from build123d import *

# Parameters (mm, degrees)
BOSS_EXTRUDE1_DEPTH   = 42.37
SKETCH2_R             = 7.45
BOSS_EXTRUDE2_DEPTH   = 1.28
BOSS_EXTRUDE3_DEPTH   = 13.58
SKETCH4_W             = 4.9
SKETCH4_H             = 11.6
BOSS_EXTRUDE4_DEPTH   = 3
M2_TAPPED_HOLE1_D     = 1.6
M2_TAPPED_HOLE1_DEPTH = 4
M2_TAPPED_HOLE1_TIP   = 0.480688495


with BuildPart() as part:
    # Sketch1 → Boss-Extrude1 (new body)
    with BuildSketch(Plane.XY):
        with BuildLine():
            Line((-8, -10), (8, -10))
            ThreePointArc((8, -10), (9.414213562, -9.414213562), (10, -8))
            Line((10, -8), (10, 8))
            ThreePointArc((10, 8), (9.414213562, 9.414213562), (8, 10))
            Line((8, 10), (-8, 10))
            ThreePointArc((-8, 10), (-9.414213562, 9.414213562), (-10, 8))
            Line((-10, 8), (-10, -8))
            ThreePointArc((-10, -8), (-9.414213562, -9.414213562), (-8, -10))
        make_face()
    extrude(amount=BOSS_EXTRUDE1_DEPTH)

    # Sketch2 → Boss-Extrude2 (add)
    with BuildSketch(Plane.XY.offset(42.37)):
        with Locations(Location((0, 0, 0), (0, 0, 180))):
            Circle(SKETCH2_R)
    extrude(amount=BOSS_EXTRUDE2_DEPTH)

    # Sketch3 → Boss-Extrude3 (add)
    with BuildSketch(Plane.XY.offset(43.65)):
        with BuildLine():
            Line((-1.5, 1.322875656), (-1.5, -1.322875656))
            ThreePointArc((-1.5, -1.322875656), (2, 0), (-1.5, 1.322875656))
        make_face()
    extrude(amount=BOSS_EXTRUDE3_DEPTH)

    # Sketch4 → Boss-Extrude4 (add)
    with BuildSketch(Plane.ZY.offset(10)):
        with Locations((5.45, 0)):
            Rectangle(SKETCH4_W, SKETCH4_H)
    extrude(amount=BOSS_EXTRUDE4_DEPTH)

    # M2 Tapped Hole1
    with Locations(Plane.XY.offset(42.37)):
        with Locations((-8, -8), (8, -8), (8, 8), (-8, 8)):
            Hole(M2_TAPPED_HOLE1_D / 2, depth=M2_TAPPED_HOLE1_DEPTH)
            with Locations((0, 0, -(M2_TAPPED_HOLE1_DEPTH + M2_TAPPED_HOLE1_TIP / 2))):  # 118° drill point
                Cone(0, M2_TAPPED_HOLE1_D / 2, M2_TAPPED_HOLE1_TIP, mode=Mode.SUBTRACT)


solid = part.part
Input: part model. Units: mm. Frame: model coordinates. A direction names the side the tool comes from. Coordinates: 2 decimals unless noted, no trailing zeros. Write each loop counter-clockwise with the first axis right and the second up, starting at its lowest first coordinate (ties: lowest second). Pieces come first, ordered by that corner, then holes. Notation, with made-up numbers: M -11.5,24.25 L 41.5,24.25 A16 cw 41.5,41.25 Z; hole C 50.25,26.25 d1. An arc over 180 degrees is marked long. Answer as a JSON object with one key per item and string values. Group by question number.
(1) Section C-C on x = -5. Output: boundary loops of the cut face in (y, z).
(2) Section D-D on y = -4.75. Output: boundary loops of the cut face in (x, z), plus the area to 3 significant figures.
(3) Mould query, pull axis Y, two halves, no side actions, for faces 1 (the face through (-11, 0, 7.9)), 2 (the face through (-9.4, 9.43, 20.89)), 3 (the face through (8.59, 8.54, 40.34)), 4 (the face through (-8.018, -7.862, 37.973)). Classes: pulls with the +Y half, pulls with the -Y half, needs draft (parallel to the pull), parting line crosses it, or undercut.
(4) Section A-A on z = 29. Output: boundary loops of the cut face in (x, y), plus the area to 3 significant figures.
(5) Ray query, line 1 along X through (y, z) = (8, 42); line 2 along Z through (x, y) = (-10.25, -3.5). Return the intervals inside material, ascending. Write a range as [from, to].
(6) Set-up query: faces 5 (the face through (-11, 0, 3)), 6 (the face through (-7.2, -8, 40.3)), 7 (the face through (-13, 0, 5)). Return all of +Z, -Z, +X, -X, +Y, -Y with unobstructed straight access to the full face (end or side cutting, diameter ignored); none if empty.
(7) Section B-B on y = 0. Output: boundary loops of the cut face in (x, z).
(8) Contact query for flat-ended pins moving along their axis: P1, Ø10, axis at y = -4, z = 27.5, coming from the -X side; P2, Ø2, axis at y = 0, z = 48, coming from the -X side; P3, Ø7.5, axis at x = 1, y = -3, coming from the +Z side; P4, Ø2.5, axis at x = -11.5, y = 2.5, coming from the -Z side. Output: stop coordinate, or through.
Result set:
{
 "1": {"outline": "M -10,0 L 10,0 L 10,42.37 L 5.52,42.37 L 5.52,43.65 L -5.52,43.65 L -5.52,42.37 L -10,42.37 Z"},
 "2": {"outline": "M -13,3 L -10,3 L -10,0 L 10,0 L 10,42.37 L 5.74,42.37 L 5.74,43.65 L -5.74,43.65 L -5.74,42.37 L -10,42.37 L -10,7.9 L -13,7.9 Z", "area": "877 mm2"},
 "3": {"face 1": "needs draft", "face 2": "pulls with the +Y half", "face 3": "undercut", "face 4": "undercut"},
 "4": {"outline": "M -10,-8 A2 ccw -8,-10 L 8,-10 A2 ccw 10,-8 L 10,8 A2 ccw 8,10 L -8,10 A2 ccw -10,8 Z", "area": "397 mm2"},
 "5": {"line 1": "x = [-10, -8.8], [-7.2, 7.2], [8.8, 10]", "line 2": "z = [3, 7.9]"},
 "6": {"face 5": "-Z, -X, +Y, -Y", "face 6": "+Z", "face 7": "+Z, -Z, -X, +Y, -Y"},
 "7": {"outline": "M -13,3 L -10,3 L -10,0 L 10,0 L 10,42.37 L 7.45,42.37 L 7.45,43.65 L 2,43.65 L 2,57.23 L -1.5,57.23 L -1.5,43.65 L -7.45,43.65 L -7.45,42.37 L -10,42.37 L -10,7.9 L -13,7.9 Z"},
 "8": {"P1": "stops at x = -10", "P2": "stops at x = -1.5", "P3": "stops at z = 57.23", "P4": "stops at z = 3"}
}
